Work out the finished part from the listing and answer in its coordinate system (mm). Face numbers are marked on the shaded views. A direction names the side the tool comes from. Coordinates: 2 decimals unless noted, no trailing zeros. Write each loop counter-clockwise with the first axis right and the second up, starting at its lowest first coordinate (ties: lowest second). Pieces come first, ordered by that corner, then holes. Notation, with made-up numbers: M 24,45.25 L 57,45.25 A19 ccw 57,65.25 Z; hole C 28.5,67.25 d10. An arc over 180 degrees is marked long. Answer as CSV lines item,"result". Start each with the question number.
(1) A cutting plane is placed at B-B on y = 31.75. Give the vertices of the cut face in (x, z), then the cut area to 3 significant figures.
(2) Find the intervals of material crossed by L1, parallel to X at y = 31.5, z = -125.5; L2, parallel to Y at x = -22.5, z = -152.5; L3, parallel to X at y = -71, z = 3.5, in increasing order. Write a range as [from, to].
(3) A cutting plane is placed at A-A on x = -63.5. Give the vertices of the cut face in (y, z), then the cut area to 3 significant figures.
(4) For the marked faces 1, 2 and 3, determine the directions among +Z, -Z, +X, -X, +Y, -Y from which every point of the face is accessible in a straight line to the end or side of a thin tool.
(5) A cutting plane is placed at D-D on z = -67. Give the vertices of the cut face in (x, y), then the cut area to 3 significant figures.
(6) A cutting plane is placed at C-C on z = -173.5. Give the vertices of the cut face in (x, y), then the cut area to 3 significant figures.
(7) Flat-ended cylindrical pins translate along their axes: P1, Ø6, axis at y = 222, z = -9.5, coming from the -X side; P2, Ø2, axis at x = -16, y = -53, coming from the +Z side; P3, Ø10, axis at y = 92.5, z = 12, coming from the +X side. Find the tip coordinate at first contact, or state that the pin passes through.
from build123d import *

# Parameters (mm, degrees)
SKETCH1_W                = 251.968
SKETCH1_H                = 336.042
BOSS_EXTRUDE1_DEPTH      = 63.5
SKETCH2_R                = 125.984
BOSS_EXTRUDE2_DEPTH      = 96.52
BOSS_EXTRUDE2_DEPTH_BACK = 274.32
SKETCH4_R                = 26.797
BOSS_EXTRUDE7_DEPTH      = 25.4


with BuildPart() as part:
    # Sketch1 → Boss-Extrude1 (new body)
    with BuildSketch(Plane(origin=(0, 0, 0), x_dir=(1, 0, 0), z_dir=(0, 1, 0))):
        with Locations((0, 42.037)):
            Rectangle(SKETCH1_W, SKETCH1_H)
    extrude(amount=BOSS_EXTRUDE1_DEPTH)

    # Sketch2 → Boss-Extrude2 (add, two sides)
    with BuildSketch(Plane.XZ) as boss_extrude2_sk:
        Circle(SKETCH2_R)
    extrude(amount=BOSS_EXTRUDE2_DEPTH)
    extrude(boss_extrude2_sk.sketch, amount=-BOSS_EXTRUDE2_DEPTH_BACK)

    # Sketch4 → Boss-Extrude7 (add)
    with BuildSketch(Plane(origin=(125.984, 0, 0), x_dir=(0, 0, -1), z_dir=(1, 0, 0))):
        with Locations((0, 31.75)):
            Circle(SKETCH4_R)
    extrude(amount=BOSS_EXTRUDE7_DEPTH)


solid = part.part
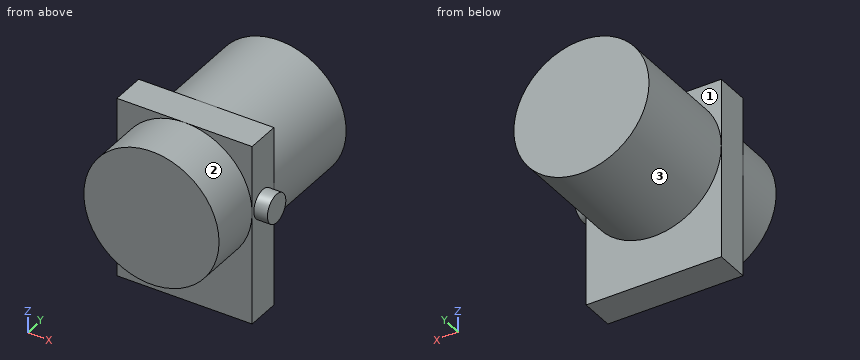
Here are the results:
1,outline,"M -125.98,-210.06 L 125.98,-210.06 L 125.98,-26.8 L 151.38,-26.8 L 151.38,26.8 L 125.98,26.8 L 125.98,125.98 L -125.98,125.98 Z"
1,area,"86,000 mm^2"
2,L1,"x = [-125.98, 125.98]"
2,L2,"y = [0, 63.5]"
2,L3,"x = [-125.94, 125.94]"
3,outline,"M -96.52,-108.81 L 0,-108.81 L 0,-210.06 L 63.5,-210.06 L 63.5,-108.81 L 274.32,-108.81 L 274.32,108.81 L 63.5,108.81 L 63.5,125.98 L 0,125.98 L 0,108.81 L -96.52,108.81 Z"
3,area,"88,200 mm^2"
4,face 1,"+Z, -X, +Y"
4,face 2,"-Y"
4,face 3,"+Y"
5,outline,"M -125.98,0 L -106.69,0 L -106.69,-96.52 L 106.69,-96.52 L 106.69,0 L 125.98,0 L 125.98,63.5 L 106.69,63.5 L 106.69,274.32 L -106.69,274.32 L -106.69,63.5 L -125.98,63.5 Z"
5,area,"81,600 mm^2"
6,outline,"M -125.98,0 L 125.98,0 L 125.98,63.5 L -125.98,63.5 Z"
6,area,"16,000 mm^2"
7,P1,"stops at x = -125.82"
7,P2,"stops at z = 125.09"
7,P3,"stops at x = 125.79"
